Geometry: final body of the model. Coordinates: model frame, mm. A direction names the side the tool comes from. Give positions to 0.01 mm unless a question says otherwise; leave off trailing zeros. Loops run counter-clockwise (first coordinate to the right, second up) from the corner with the lowest first, then second, coordinate; pieces in that order, holes last.
from build123d import *

# Parameters (mm, degrees)
F0_R     = 1.7272
F0_R_2   = 3.175
F1_DEPTH = 9.525
F3_DEPTH = 3.175


with BuildPart() as f1:
    # F0 (on Top) → F1 (new body)
    with BuildSketch(Plane.XY):
        with BuildLine():
            Line((-4.7625, 9.895144), (-4.7625, 6.807021))
            ThreePointArc((-4.7625, 6.807021), (-8.307644, 0), (-4.7625, -6.807021))
            Line((-4.7625, -6.807021), (-4.7625, -9.895144))
            ThreePointArc((-4.7625, -9.895144), (0, -14.657644), (4.7625, -9.895144))
            Line((4.7625, -9.895144), (4.7625, -6.807021))
            ThreePointArc((4.7625, -6.807021), (8.307644, 0), (4.7625, 6.807021))
            Line((4.7625, 6.807021), (4.7625, 9.895144))
            ThreePointArc((4.7625, 9.895144), (0, 14.657644), (-4.7625, 9.895144))
        make_face()
        with Locations((0, -9.895144)):
            Circle(F0_R, mode=Mode.SUBTRACT)
        Circle(F0_R_2, mode=Mode.SUBTRACT)
        with Locations((0, 9.895144)):
            Circle(F0_R, mode=Mode.SUBTRACT)
    extrude(amount=F1_DEPTH)

    # F2 (on face) → F3 (cut)
    with BuildSketch(Plane(origin=(0, 0, 0), x_dir=(1, 0, 0), z_dir=(0, 0, -1))):
        Polygon((-2.566322, 4.445), (-5.132644, 0), (-2.566322, -4.445), (2.566322, -4.445), (5.132644, 0), (2.566322, 4.445), align=None)
    extrude(amount=-F3_DEPTH, mode=Mode.SUBTRACT)


solid = f1.part
Item 1: Section query C-C on y = -2. Return loops of the section in (x, z) (3 decimals).
Values follow:
outline: (-8.063, 0) - (-3.978, 0) - (-3.978, 3.175) - (-2.466, 3.175) - (-2.466, 9.525) - (-8.063, 9.525) - close; (2.466, 3.175) - (3.978, 3.175) - (3.978, 0) - (8.063, 0) - (8.063, 9.525) - (2.466, 9.525) - close
Item 2: Section query B-B on x = 0. Return loops of the section in (y, z) (3 decimals).
Values follow:
outline: (-14.658, 0) - (-11.622, 0) - (-11.622, 9.525) - (-14.658, 9.525) - close; (-8.168, 0) - (-4.445, 0) - (-4.445, 3.175) - (-3.175, 3.175) - (-3.175, 9.525) - (-8.168, 9.525) - close; (3.175, 3.175) - (4.445, 3.175) - (4.445, 0) - (8.168, 0) - (8.168, 9.525) - (3.175, 9.525) - close; (11.622, 0) - (14.658, 0) - (14.658, 9.525) - (11.622, 9.525) - close
Item 3: Section query D-D on x = -3.75. Return loops of the section in (y, z) (3 decimals), plus the area to 3 significant figures.
Values follow:
outline: (-12.831, 0) - (-2.395, 0) - (-2.395, 3.175) - (2.395, 3.175) - (2.395, 0) - (12.831, 0) - (12.831, 9.525) - (-12.831, 9.525) - close
area: 229 mm2
Item 4: Set-up query: faces 1 (the face through (4.762, 8, 5)), 2 (the face through (3.87, -2.19, 1.57)), 3 (the face through (-4.762, -8, 5)), 4 (the face through (-0.1, 3.5, 9.525)). Return all of +Z, -Z, +X, -X, +Y, -Y with unobstructed straight access to the full face (end or side cutting, diameter ignored); none if empty.
Values follow:
face 1: +Z, -Z, +X, +Y
face 2: -Z
face 3: +Z, -Z, -X, -Y
face 4: +Z, +X, -X, +Y, -Y
Item 5: Draft query along Y for faces 5 (the face through (8.307, -0.112, 4.696)), 6 (the face through (-0.69, -3.1, 6.31)), 7 (the face through (4.762, -8, 5)). Return one class per face: +Y half, -Y half, draft (parallel to the pull), parting line (faces both ways), or undercut.
Values follow:
face 5: parting line
face 6: undercut
face 7: draft
Item 6: Section query A-A on z = 2.5. Return loops of the section in (x, y) (1 decimal).
Values follow:
outline: (-4.8, -9.9) arc R4.8 ccw to (4.8, -9.9) - (4.8, -6.8) arc R8.3 ccw to (4.8, 6.8) - (4.8, 9.9) arc R4.8 ccw to (-4.8, 9.9) - (-4.8, 6.8) arc R8.3 ccw to (-4.8, -6.8) - close; hole (-5.1, 0) - (-2.6, -4.4) - (2.6, -4.4) - (5.1, 0) - (2.6, 4.4) - (-2.6, 4.4) - close; hole circle Ø3.5 at (0, -9.9); hole circle Ø3.5 at (0, 9.9)
Item 7: Pin query (flat end, axial travel): pin 1 (4 mm diameter, centred on y = -11, z = 2, fed in from +X); pin 2 (2 mm diameter, centred on x = 2, z = 1, fed in from +Y); pin 3 (1.6 mm diameter, centred on x = 1, z = 1, fed in from +Y). Return the tip coordinate at first contact, or that it passes through.
Values follow:
pin 1: stops at x = 4.76
pin 2: stops at y = 14.55
pin 3: stops at y = 14.65
Item 8: Ray query, probe 1 along Y at (x, z) = (0, 7) (3 decimals); probe 2 along X at (y, z) = (0, 7.5) (3 decimals); probe 3 along X at (y, z) = (10, 4.5). Return the intervals inside material, ascending.
Values follow:
probe 1: y = -14.658 to -11.622, -8.168 to -3.175, 3.175 to 8.168, 11.622 to 14.658
probe 2: x = -8.308 to -3.175, 3.175 to 8.308
probe 3: x = -4.76 to -1.72, 1.72 to 4.76
